from build123d import *

# Parameters (mm, degrees)
SKETCH1_W           = 28
SKETCH1_H           = 20
BOSS_EXTRUDE1_DEPTH = 4.8
SKETCH2_W           = 20
SKETCH2_H           = 28
BOSS_EXTRUDE2_DEPTH = 4.8
CUT_EXTRUDE1_DEPTH  = 5.8
CUT_EXTRUDE2_DEPTH  = 5.8
BOSS_EXTRUDE3_DEPTH = 3
BOSS_EXTRUDE4_DEPTH = 3


with BuildPart() as part:
    # Sketch1 → Boss-Extrude1 (new body)
    with BuildSketch(Plane(origin=(0, 0, 0), x_dir=(1, 0, 0), z_dir=(0, 1, 0))):
        Rectangle(SKETCH1_W, SKETCH1_H)
    extrude(amount=BOSS_EXTRUDE1_DEPTH)

    # Sketch2 → Boss-Extrude2 (add)
    with BuildSketch(Plane.ZY.offset(14)):
        with Locations((0, 14)):
            Rectangle(SKETCH2_W, SKETCH2_H)
    extrude(amount=-BOSS_EXTRUDE2_DEPTH)

    # Sketch3 → Cut-Extrude1 (cut, through all)
    with BuildSketch(Plane(origin=(-9.2, 0, 0), x_dir=(0, 0, -1), z_dir=(1, 0, 0))):
        with BuildLine():
            Line((3, 18.4), (3, 14.4))
            ThreePointArc((3, 14.4), (0, 11.4), (-3, 14.4))
            Line((-3, 14.4), (-3, 18.4))
            ThreePointArc((-3, 18.4), (0, 21.4), (3, 18.4))
        make_face()
    extrude(amount=-CUT_EXTRUDE1_DEPTH, mode=Mode.SUBTRACT)

    # Sketch4 → Cut-Extrude2 (cut, through all)
    with BuildSketch(Plane(origin=(0, 4.8, 0), x_dir=(1, 0, 0), z_dir=(0, 1, 0))):
        with BuildLine():
            Line((0.4, 3), (4.4, 3))
            ThreePointArc((4.4, 3), (7.4, 0), (4.4, -3))
            Line((4.4, -3), (0.4, -3))
            ThreePointArc((0.4, -3), (-2.6, 0), (0.4, 3))
        make_face()
    extrude(amount=-CUT_EXTRUDE2_DEPTH, mode=Mode.SUBTRACT)

    # Sketch5 → Boss-Extrude3 (add)
    with BuildSketch(Plane.XY.offset(10)):
        Polygon((-9.2, 28), (14, 4.8), (-9.2, 4.8), align=None)
    extrude(amount=-BOSS_EXTRUDE3_DEPTH)

    # Sketch6 → Boss-Extrude4 (add)
    with BuildSketch(Plane(origin=(0, 0, -10), x_dir=(-1, 0, 0), z_dir=(0, 0, -1))):
        Polygon((9.2, 28), (9.2, 4.8), (-14, 4.8), align=None)
    extrude(amount=-BOSS_EXTRUDE4_DEPTH)


solid = part.part
Can you work these out from the model? Positions are in its coordinate system, mm. A direction names the side the tool comes from. Round coordinates to 2 decimals unless told otherwise and drop trailing zeros. Write each loop counter-clockwise with the first axis right and the second up, starting at its lowest first coordinate (ties: lowest second). Pieces come first, ordered by that corner, then holes. Notation, with made-up numbers: M 37.25,-4 L 66.25,-4 A21 ccw 66.25,12 Z; hole C 78.25,17 d8. An arc over 180 degrees is marked long. Use CSV: the item, a comma, the result in double quotes.
(1) I'm going to push flat-ended pins straight in: pin 1 (12 mm diameter, centred on x = 10, z = 6.5, fed in from +Y); pin 2 (4 mm diameter, centred on x = 5.5, z = 3, fed in from +Y). Where does each tip first touch, or does it pass through?
Check values:
pin 1,"y = 14.78"
pin 2,"y = 4.8"
(2) Imagine slicing it at D-D (y = 6.75). Write out the boundary of the cut face in (x, z).
Check values:
outline,"M -14,-10 L 12.05,-10 L 12.05,-7 L -9.2,-7 L -9.2,7 L 12.05,7 L 12.05,10 L -14,10 Z"
(3) We'd pull the mould along Y, two halves only. Please class faces 6 (the cylindrical face through (-11.6, 21.4, 0.1)), 7 (the flat face through (-12, 28, 0)), 8 (the flat face through (-9.2, 16.6, -3.2)), 9 (the flat face through (-3, 0, 0)): +Y half, -Y half, draft (parallel to the pull), parting line (faces both ways), or undercut.
Check values:
face 6,"undercut"
face 7,"+Y half"
face 8,"draft"
face 9,"-Y half"
(4) Imagine slicing it at B-B (y = 3.5). Write out the boundary of the cut face in (x, z).
Check values:
outline,"M -14,-10 L 14,-10 L 14,10 L -14,10 Z; hole M 0.4,-3 L 4.4,-3 A3 ccw 4.4,3 L 0.4,3 A3 ccw Z"
(5) Imagine slicing it at A-A (z = 0). Write out the boundary of the cut face in (x, y), plus the area to 3 significant figures.
Check values:
outline,"M -14,0 L -2.6,0 L -2.6,4.8 L -9.2,4.8 L -9.2,11.4 L -14,11.4 Z; M -14,21.4 L -9.2,21.4 L -9.2,28 L -14,28 Z; M 7.4,0 L 14,0 L 14,4.8 L 7.4,4.8 Z"
area,"150 mm^2"
(6) On a 3-axis mill with a long thin cutter (end or side, diameter ignored), from which of +Z, -Z, +X, -X, +Y, -Y can I reach the whole of each face in a straight line? I mean faces 1 (the cylindrical face through (7.4, 2.4, -0.1)), 2 (the flat face through (-14, 11, 0)), 3 (the flat face through (-3, 11, -10)), 4 (the flat face through (2.2, 4.8, -3.2)), 5 (the flat face through (-12, 16, -3)). Say none if no direction works.
Check values:
face 1,"+Y, -Y"
face 2,"+Z, -Z, -X, +Y, -Y"
face 3,"-Z, +X, -X, +Y, -Y"
face 4,"+X, +Y"
face 5,"+X, -X"
(7) Imagine slicing it at C-C (x = 1.25). Write out the boundary of the cut face in (y, z).
Check values:
outline,"M 0,-10 L 17.55,-10 L 17.55,-7 L 4.8,-7 L 4.8,-3 L 0,-3 Z; M 0,3 L 4.8,3 L 4.8,7 L 17.55,7 L 17.55,10 L 0,10 Z"
(8) I need wall thicknesses on line 1 along Z through (x, y) = (-0.75, 19.25); line 2 along X through (y, z) = (26.25, 4.5); line 3 along Y through (x, z) = (12.5, 0). Which ranges of each line are inside material? Lowest first, please.
Check values:
line 1,"-10 to -7, 7 to 10"
line 2,"-14 to -9.2"
line 3,"0 to 4.8"
